Build history of the part. All positions in model axes, mm. Give positions to 0.01 mm unless a question says otherwise; leave off trailing zeros. Write each loop counter-clockwise with the first axis right and the second up, starting at its lowest first coordinate (ties: lowest second). Pieces come first, ordered by that corner, then holes. Notation, with made-up numbers: (-21, 59.25) -> (37, 59.25) arc R30 cw to (37, 81.25) -> close; hole circle Ø10 at (63, 56.5). An arc over 180 degrees is marked (long way). Put each result on its own line as item: value.
from build123d import *

# Parameters (mm, degrees)
SKETCH1_R           = 14
BOSS_EXTRUDE1_DEPTH = 3


with BuildPart() as part:
    # Sketch1 → Boss-Extrude1 (new body)
    with BuildSketch(Plane(origin=(0, 0, 0), x_dir=(0, 0, -1), z_dir=(1, 0, 0))):
        Polygon((-66.6, -12.5), (-66.6, -20), (66.6, -20), (66.6, -12.5), (69.6, -12.5), (69.6, 12.5), (66.6, 12.5), (66.6, 20), (50, 20), (50, 23), (25, 23), (25, 20), (-25, 20), (-25, 23), (-50, 23), (-50, 20), (-66.6, 20), (-66.6, 12.5), (-69.6, 12.5), (-69.6, -12.5), align=None)
        with Locations((-48.6, 0)):
            Circle(SKETCH1_R, mode=Mode.SUBTRACT)
        with Locations((-16.6, 0)):
            Circle(SKETCH1_R, mode=Mode.SUBTRACT)
        with Locations((16.6, 0)):
            Circle(SKETCH1_R, mode=Mode.SUBTRACT)
        with Locations((48.6, 0)):
            Circle(SKETCH1_R, mode=Mode.SUBTRACT)
    extrude(amount=BOSS_EXTRUDE1_DEPTH)


solid = part.part
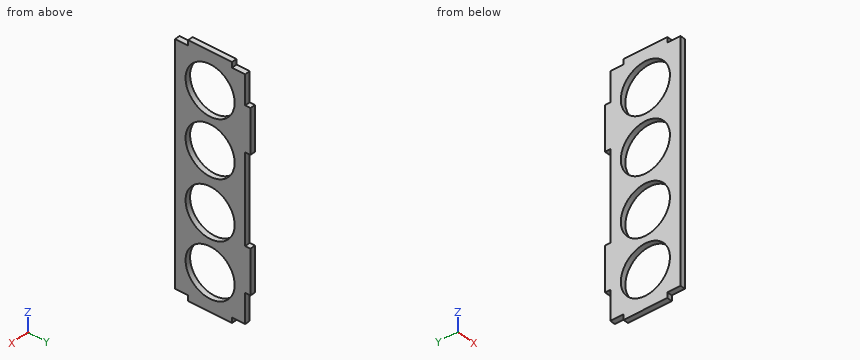
1) Wall check: L1, parallel to Z at x = 0.8, y = 8.5; L2, parallel to Z at x = 1.7, y = -2; L3, parallel to Y at x = 1, z = -16.6. Give the ranges that are in metal, low to high.
Filled sheet:
L1: -69.6 to -59.72, -37.48 to -27.72, -5.48 to 5.48, 27.72 to 37.48, 59.72 to 69.6
L2: -69.6 to -62.46, -34.74 to -30.46, -2.74 to 2.74, 30.46 to 34.74, 62.46 to 69.6
L3: -20 to -14, 14 to 20
2) Pin check, flat tips, straight feed: pin 1 (0.9 mm diameter, centred on x = 1.5, y = 22, fed in from +Z); pin 2 (0.9 mm diameter, centred on x = 1, y = -14.5, fed in from -Z); pin 3 (1.5 mm diameter, centred on x = 1, y = 21, fed in from -Z). Stop position of each tip, or through.
Filled sheet:
pin 1: z = 50
pin 2: z = -66.6
pin 3: z = -50
3) Slice it at A-A (z = -48.6). Write the cut outline in (x, y), plus the area to 3 significant figures.
Filled sheet:
outline: (0, -20) -> (3, -20) -> (3, -14) -> (0, -14) -> close; (0, 14) -> (3, 14) -> (3, 23) -> (0, 23) -> close
area: 45.0 mm2
4) Slice it at C-C (x = 0.6). Write the cut outline in (y, z), plus the area to 4 significant figures.
Filled sheet:
outline: (-20, -66.6) -> (-12.5, -66.6) -> (-12.5, -69.6) -> (12.5, -69.6) -> (12.5, -66.6) -> (20, -66.6) -> (20, -50) -> (23, -50) -> (23, -25) -> (20, -25) -> (20, 25) -> (23, 25) -> (23, 50) -> (20, 50) -> (20, 66.6) -> (12.5, 66.6) -> (12.5, 69.6) -> (-12.5, 69.6) -> (-12.5, 66.6) -> (-20, 66.6) -> close; hole circle Ø28 at (0, -48.6); hole circle Ø28 at (0, -16.6); hole circle Ø28 at (0, 16.6); hole circle Ø28 at (0, 48.6)
area: 3,165 mm2
5) Slice it at B-B (y = 0). Write the cut outline in (x, z), plus the area to 3 significant figures.
Filled sheet:
outline: (0, -69.6) -> (3, -69.6) -> (3, -62.6) -> (0, -62.6) -> close; (0, -34.6) -> (3, -34.6) -> (3, -30.6) -> (0, -30.6) -> close; (0, -2.6) -> (3, -2.6) -> (3, 2.6) -> (0, 2.6) -> close; (0, 30.6) -> (3, 30.6) -> (3, 34.6) -> (0, 34.6) -> close; (0, 62.6) -> (3, 62.6) -> (3, 69.6) -> (0, 69.6) -> close
area: 81.6 mm2
6) Slice it at D-D (z = 16.6). Write the cut outline in (x, y), plus the area to 3 significant figures.
Filled sheet:
outline: (0, -20) -> (3, -20) -> (3, -14) -> (0, -14) -> close; (0, 14) -> (3, 14) -> (3, 20) -> (0, 20) -> close
area: 36.0 mm2
